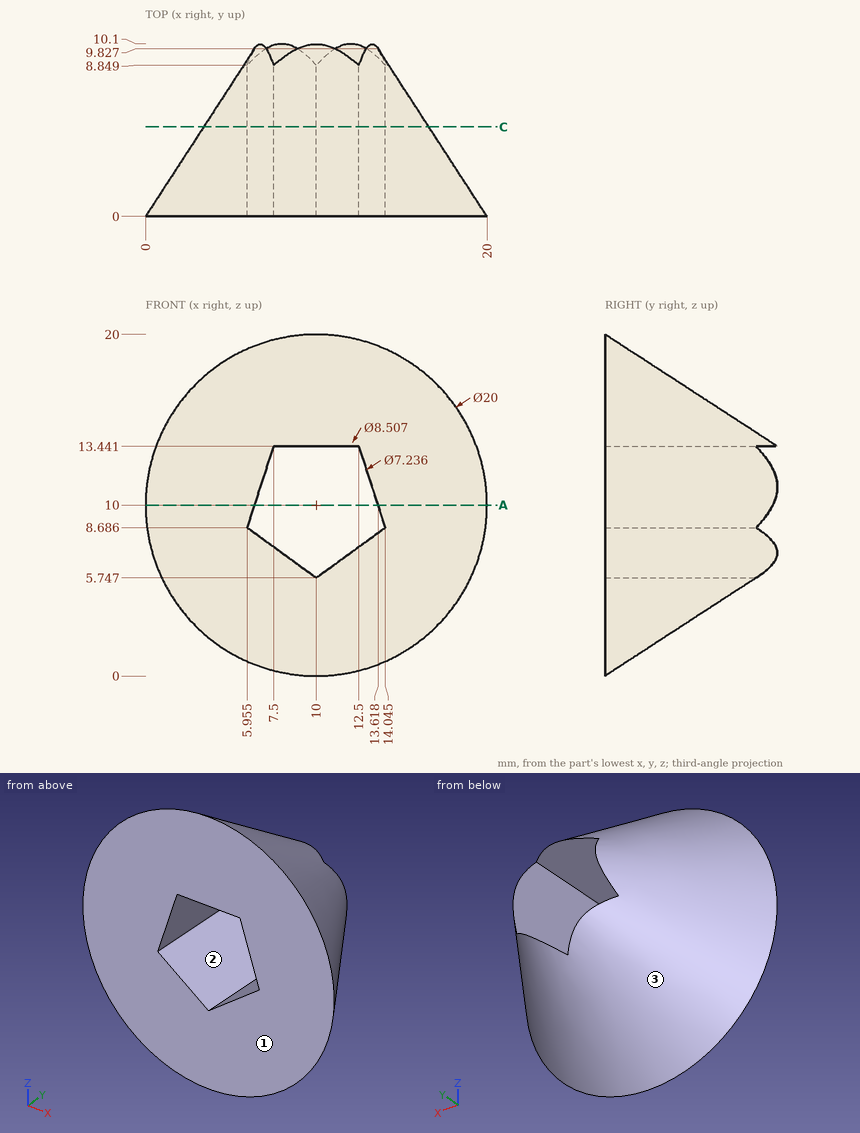
Part print with two shaded views. Sizes in mm from the minimum x, y, z corner. Give positions to 0.01 mm unless a question says otherwise; leave off trailing zeros. Order: outer loops, then holes, each group sorted by start corner. A loop starts at its lowest first (then second) coordinate and runs counter-clockwise, first axis right, second up. Notation, with made-up numbers: M 2.25,-11.75 L 15.25,-11.75 A21 cw 15.25,23.25 Z; hole C -6,81.5 d10. An arc over 180 degrees is marked long. Write item = value, one per line.
Q1. Cut at A-A, the plane z = 10. List the corners of the cut face in (x, y).
Derived:
outline = M 0,0 L 6.38,0 L 6.38,9.83 Z; M 13.62,0 L 20,0 L 13.62,9.83 Z
Q2. Cut at C-C, the plane y = 5.25. List the corners of the cut face in (x, z) (1 decimal).
Derived:
outline = C 10,10 d13.2; hole M 6,8.7 L 10,5.7 L 14,8.7 L 12.5,13.4 L 7.5,13.4 Z
Q3. Flat gauge pins, fed straight in: pin 1 (5 mm diameter, centred on x = 2.5, z = 13.5, fed in from +Y) (1 decimal); pin 2 (2.5 mm diameter, centred on x = 11, y = 2.5, fed in from -Z); pin 3 (4 mm diameter, centred on y = 3.5, z = 8, fed in from +X). Where does each tip first touch, or does it go through?
Derived:
pin_1 = 6.5
pin_2 = 0.86
pin_3 = 18.86
Q4. Two-plate mould, pull along Z, no slides. Class the marked faces 1, 2 and 3: pulls with the +Z half, pulls with the -Z half, needs draft (parallel to the pull), parting line crosses it, or undercut.
Derived:
face_1 = needs draft
face_2 = undercut
face_3 = parting line crosses it
Q5. Drill centre lines: line 1 (X direction, y = 3.5, z = 10.25) (1 decimal); line 2 (Z direction, x = 9.75, y = 8.5) (1 decimal); line 3 (X direction, y = 4, z = 10.25) (1 decimal). Where is each one in solid material? Low to high. Write a range as [from, to].
Derived:
line_1 = [2.3, 6.5], [13.5, 17.7]
line_2 = [5.5, 5.9], [13.4, 14.5]
line_3 = [2.6, 6.5], [13.5, 17.4]
